```python
from build123d import *

# Parameters (mm, degrees)
SKETCH1_W               = 29.972
SKETCH1_H               = 23.114
EXTRUDE1_DEPTH          = 11.938
CUT_EXTRUDE1_DEPTH      = 12.938
SKETCH3_W               = 2.27457
SKETCH3_H               = 7.704666667
CUT_EXTRUDE2_DEPTH      = 15.986
CUT_EXTRUDE2_DEPTH_BACK = 15.986
SKETCH4_W               = 28.3845
SKETCH4_H               = 10.3505
CUT_EXTRUDE3_DEPTH      = 0.254
SKETCH5_W               = 1.255132872
SKETCH5_H               = 4.83743
CUT_EXTRUDE4_DEPTH      = 1.524
EXTRUDE2_DEPTH          = 0.635
CUT_EXTRUDE5_DEPTH      = 12.938


with BuildPart() as part:
    # Sketch1 → Extrude1 (new body)
    with BuildSketch(Plane.XY):
        Rectangle(SKETCH1_W, SKETCH1_H)
    extrude(amount=EXTRUDE1_DEPTH)

    # Sketch2 → Cut-Extrude1 (cut, through all)
    with BuildSketch(Plane.XY.offset(11.938)):
        with BuildLine():
            Line((-9.990666667, 3.852333333), (-9.790853333, 3.852333333))
            ThreePointArc((-9.790853333, 3.852333333), (-10.010454448, 6.185541418), (-9.5329375, 8.479895833))
            Line((-9.5329375, 8.479895833), (-9.5329375, 11.504083333))
            Line((-9.5329375, 11.504083333), (-12.557125, 11.557))
            Line((-12.557125, 11.557), (12.557125, 11.557))
            Line((12.557125, 11.557), (9.5329375, 11.504083333))
            Line((9.5329375, 11.504083333), (9.5329375, 8.479895833))
            ThreePointArc((9.5329375, 8.479895833), (10.010454448, 6.185541418), (9.790853333, 3.852333333))
            Line((9.790853333, 3.852333333), (9.990666667, 3.852333333))
            ThreePointArc((9.990666667, 3.852333333), (0, -6.138333333), (-9.990666667, 3.852333333))
        make_face()
    extrude(amount=-CUT_EXTRUDE1_DEPTH, mode=Mode.SUBTRACT)

    # Sketch3 → Cut-Extrude2 (cut, two sides)
    with BuildSketch(Plane(origin=(0, 0, 0), x_dir=(0, 0, -1), z_dir=(1, 0, 0))) as cut_extrude2_sk:
        with Locations((-10.800715, 7.704666667)):
            Rectangle(SKETCH3_W, SKETCH3_H)
        with Locations((-1.137285, 7.704666667)):
            Rectangle(SKETCH3_W, SKETCH3_H)
    extrude(amount=CUT_EXTRUDE2_DEPTH, mode=Mode.SUBTRACT)
    extrude(cut_extrude2_sk.sketch, amount=-CUT_EXTRUDE2_DEPTH_BACK, mode=Mode.SUBTRACT)

    # Sketch4 → Cut-Extrude3 (cut)
    with BuildSketch(Plane.XZ.offset(11.557)):
        with Locations((0, 5.969)):
            Rectangle(SKETCH4_W, SKETCH4_H)
    extrude(amount=-CUT_EXTRUDE3_DEPTH, mode=Mode.SUBTRACT)

    # Sketch5 → Cut-Extrude4 (cut)
    with BuildSketch(Plane(origin=(0, 11.557, 0), x_dir=(1, 0, 0), z_dir=(0, 1, 0))):
        with Locations((-14.358433564, -5.969)):
            Rectangle(SKETCH5_W, SKETCH5_H)
        with Locations((14.358433564, -5.969)):
            Rectangle(SKETCH5_W, SKETCH5_H)
    extrude(amount=-CUT_EXTRUDE4_DEPTH, mode=Mode.SUBTRACT)

    # Sketch6 → Cut-Revolve1 (revolve, cut)
    with BuildSketch(Plane(origin=(0, 0, 5.969), x_dir=(-1, 0, 0), z_dir=(0, 0, -1)), mode=Mode.PRIVATE) as cut_revolve1_sk:
        Polygon((2.54, -11.303), (0, -11.303), (0, -6.223), (4.953, -6.223), (4.953, -8.763), (2.54, -8.763), align=None)
    revolve(cut_revolve1_sk.sketch.rotate(Axis((0, 0, 5.969), (0, -1, 0)), 270), axis=Axis((0, 0, 5.969), (0, -1, 0)), mode=Mode.SUBTRACT)  # turned: the seam where the file's is

    # Sketch7 → Extrude2 (add, symmetric)
    with BuildSketch(Plane(origin=(0, 0, 5.969), x_dir=(-1, 0, 0), z_dir=(0, 0, -1))):
        with BuildLine():
            Line((4.047558738, -4.067217721), (7.45308183, -1.000870956))
            Line((7.45308183, -1.000870956), (8.209636208, -1.841109717))
            ThreePointArc((8.209636208, -1.841109717), (6.685060845, -3.572178903), (4.804113117, -4.907456482))
            Line((4.804113117, -4.907456482), (4.047558738, -4.067217721))
        make_face()
        with BuildLine():
            Line((-4.047558738, -4.067217721), (-4.804113117, -4.907456482))
            ThreePointArc((-4.804113117, -4.907456482), (-6.685060845, -3.572178903), (-8.209636208, -1.841109717))
            Line((-8.209636208, -1.841109717), (-7.45308183, -1.000870956))
            Line((-7.45308183, -1.000870956), (-4.047558738, -4.067217721))
        make_face()
    extrude(amount=EXTRUDE2_DEPTH, both=True)

    # Sketch8 → Cut-Extrude5 (cut, through all)
    with BuildSketch(Plane.XY):
        Polygon((-9.5329375, 11.538527778), (-11.5014375, 11.538527778), (-9.5329375, 8.935027778), align=None)
        Polygon((9.5329375, 11.538527778), (11.5014375, 11.538527778), (9.5329375, 8.935027778), align=None)
    extrude(amount=CUT_EXTRUDE5_DEPTH, mode=Mode.SUBTRACT)


solid = part.part
```
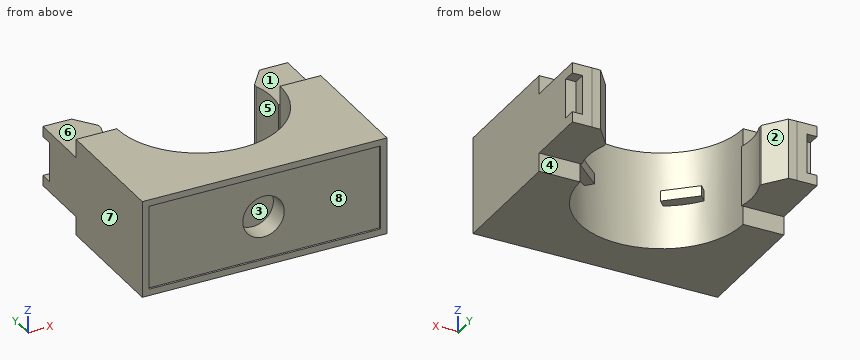
The model under review builds one solid part; all positions refer to its coordinate system, in mm. Face numbers are marked on the shaded views. A direction names the side the tool comes from. Give positions to 0.01 mm unless a question says otherwise; leave off trailing zeros. Loops run counter-clockwise (first coordinate to the right, second up) from the corner with the lowest first, then second, coordinate; pieces in that order, holes last. Notation, with made-up numbers: (4.25, 16) -> (45.25, 16) arc R23 ccw to (45.25, 46) -> close; hole circle Ø4 at (88, 56). An arc over 180 degrees is marked (long way). Use CSV: the item, a comma, the result in double quotes.
1. Consider section C-C, the plane y = -9.25. Write out the cut boundary in (x, z).
Result:
outline,"(-14.99, 0) -> (14.99, 0) -> (14.99, 11.94) -> (-14.99, 11.94) -> close; hole circle Ø5.08 at (0, 5.97)"
2. Machinability: for the marked faces 1, 2, 3, 4 and 5, which of the approach directions +Z, -Z, +X, -X, +Y, -Y give a long, thin tool a straight path to every point of the face, cutting with its end or side? Answer none if there is none.
Result:
face 1,"+Z, +X, -X, +Y"
face 2,"+Z, -Z, +Y"
face 3,"none"
face 4,"-Z, +X, -X, +Y"
face 5,"+Z, -Z"
3. To check wall thickness, follow probe 1 along X at (y, z) = (8, 4.5); probe 2 along X at (y, z) = (0, 8.5); probe 3 along Y at (x, z) = (4.5, 7). State the ranges of each line that lie inside material, in increasing order. Write a range as from..to.
Result:
probe 1,"x = -14.99..-9.69, 9.69..14.99"
probe 2,"x = -14.99..-9.22, 9.22..14.99"
probe 3,"y = -11.3..-8.76, -6.22..-5.07"
4. The part is to be moulded in two halves that separate along Z. For the marked faces 6, 7 and 8, say which applies: +Z half, -Z half, draft (parallel to the pull), parting line (faces both ways), or undercut.
Result:
face 6,"+Z half"
face 7,"draft"
face 8,"undercut"
5. Consider section B-B, the plane x = 0. Write out the cut boundary in (y, z).
Result:
outline,"(-11.56, 0) -> (-6.14, 0) -> (-6.14, 11.94) -> (-11.56, 11.94) -> (-11.56, 11.14) -> (-11.3, 11.14) -> (-11.3, 8.51) -> (-8.76, 8.51) -> (-8.76, 10.92) -> (-6.22, 10.92) -> (-6.22, 1.02) -> (-8.76, 1.02) -> (-8.76, 3.43) -> (-11.3, 3.43) -> (-11.3, 0.79) -> (-11.56, 0.79) -> close"
6. For P1, Ø0.6, axis at x = -14.5, y = 11, coming from the +Z side; P2, Ø3, axis at x = 1.5, z = 6.5, coming from the -Y side; P3, Ø0.5, axis at y = 11, z = 6.5, coming from the -X side, all flat-tipped, find the tip position at first contact; note any pin that passes through.
Result:
P1,"stops at z = 9.66"
P2,"stops at y = -11.3"
P3,"stops at x = -13.73"
7. Consider section A-A, the plane y = -5.5. Write out the cut boundary in (x, z), then the cut area to 3 significant figures.
Result:
outline,"(-14.99, 0) -> (-3.51, 0) -> (-3.51, 11.94) -> (-14.99, 11.94) -> close; (3.51, 0) -> (14.99, 0) -> (14.99, 11.94) -> (3.51, 11.94) -> close"
area,"274 mm²"
